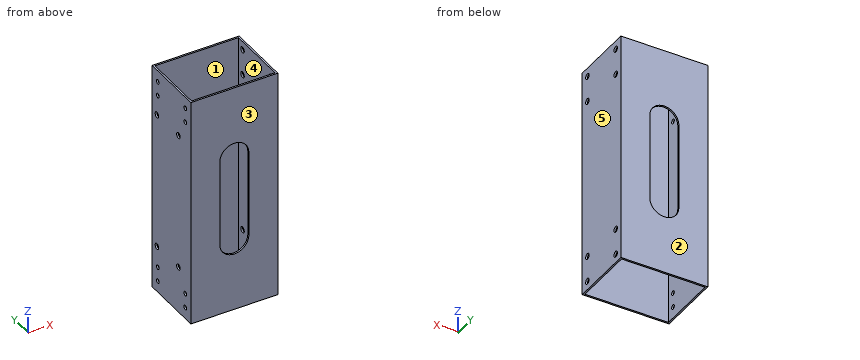
from build123d import *

# Parameters (mm, degrees)
SKETCH_1_W          = 60
SKETCH_1_H          = 45
SKETCH_1_W_2        = 57.6
SKETCH_1_H_2        = 42.6
EXTRUDE_1_DEPTH     = 80
SKETCH_4_R          = 2.025
CUT_EXTRUDE_1_DEPTH = 5
SKETCH_5_R          = 1.55
CUT_EXTRUDE_2_DEPTH = 5
SKETCH_6_R          = 2.025
CUT_EXTRUDE_3_DEPTH = 1.2
CUT_EXTRUDE_4_DEPTH = 160


with BuildPart() as part:
    # 草图1 → 凸台-拉伸1 (new body, symmetric)
    with BuildSketch(Plane.XY):
        Rectangle(SKETCH_1_W, SKETCH_1_H)
        Rectangle(SKETCH_1_W_2, SKETCH_1_H_2, mode=Mode.SUBTRACT)
    extrude(amount=EXTRUDE_1_DEPTH, both=True)

    # 草图4 → 切除-拉伸1 (cut, symmetric)
    with BuildSketch(Plane(origin=(30, 0, 0), x_dir=(0, 0, -1), z_dir=(1, 0, 0))):
        with Locations((-74, 16.5)):
            Circle(SKETCH_4_R)
        with Locations((-56, 16.5)):
            Circle(SKETCH_4_R)
        with Locations((-74, -16.5)):
            Circle(SKETCH_4_R)
        with Locations((-56, -16.5)):
            Circle(SKETCH_4_R)
    cut_extrude_1 = extrude(amount=CUT_EXTRUDE_1_DEPTH, both=True, mode=Mode.SUBTRACT)

    # 镜向1: 切除-拉伸1 across plane
    add(cut_extrude_1.mirror(Plane.XY), mode=Mode.SUBTRACT)

    # 草图5 → 切除-拉伸2 (cut, symmetric)
    with BuildSketch(Plane.ZY.offset(30)):
        with Locations((62, 16)):
            Circle(SKETCH_5_R)
        with Locations((72, 16)):
            Circle(SKETCH_5_R)
        with Locations((62, -16)):
            Circle(SKETCH_5_R)
        with Locations((72, -16)):
            Circle(SKETCH_5_R)
    cut_extrude_2 = extrude(amount=CUT_EXTRUDE_2_DEPTH, both=True, mode=Mode.SUBTRACT)

    # 镜向2: 切除-拉伸2 across plane
    add(cut_extrude_2.mirror(Plane.XY), mode=Mode.SUBTRACT)

    # 草图6 → 切除-拉伸3 (cut)
    with BuildSketch(Plane.ZY.offset(30)):
        with Locations((47.5, -8)):
            Circle(SKETCH_6_R)
        with Locations((47.5, 17)):
            Circle(SKETCH_6_R)
        with Locations((-47.5, 17)):
            Circle(SKETCH_6_R)
        with Locations((-47.5, -8)):
            Circle(SKETCH_6_R)
    extrude(amount=-CUT_EXTRUDE_3_DEPTH, mode=Mode.SUBTRACT)

    # 草图7 → 切除-拉伸4 (cut)
    with BuildSketch(Plane.XZ.offset(22.5)):
        with BuildLine():
            Line((-10, -30), (-10, 30))
            ThreePointArc((-10, 30), (0, 40), (10, 30))
            Line((10, 30), (10, -30))
            ThreePointArc((10, -30), (0, -40), (-10, -30))
        make_face()
    extrude(amount=-CUT_EXTRUDE_4_DEPTH, mode=Mode.SUBTRACT)


solid = part.part
The model under review builds one solid part; all positions refer to its coordinate system, in mm. Face numbers are marked on the shaded views. A direction names the side the tool comes from. Give positions to 0.01 mm unless a question says otherwise; leave off trailing zeros. Order: outer loops, then holes, each group sorted by start corner. A loop starts at its lowest first (then second) coordinate and runs counter-clockwise, first axis right, second up. Notation, with made-up numbers: (-36, 57) -> (-26, 57) arc R13 ccw to (-26, 61) -> close; hole circle Ø8 at (-32.5, -8.75). An arc over 180 degrees is marked (long way). Write item = value, one per line. Start each with the question number.
(1) Take a section at A-A (x = 0). Write out the cut boundary in (y, z).
(2) Draft analysis for pull direction X (two halves, no side actions). For the marked faces 3, 4 and 5, state which applies: +X half, -X half, draft (parallel to the pull), parting line (faces both ways), or undercut.
(3) Take a section at C-C (z = -52). Write out the cut boundary in (x, y).
(4) For pin 1 Ø2.5 at (y, z) = (-16, 72) entering from -X; pin 2 Ø3 at (y, z) = (-16.5, -74) entering from +X; pin 3 Ø5.5 at (y, z) = (17, -47.5) entering from -X, all flat-tipped, find the tip position at first contact; note any pin that passes through.
(5) Take a section at B-B (y = -1.5). Write out the cut boundary in (x, z).
(6) Tool access review of the marked faces 1 and 2: name each direction out of +Z, -Z, +X, -X, +Y, -Y from which nothing blocks a thin tool from reaching the whole face with its end or side.
(7) For L1, parallel to Y at x = 29, z = 56 (3 decimals); L2, parallel to X at y = 19, z = -42.5; L3, parallel to Y at x = -5, z = -55, list the stretches that pass through material, from the lowest coordinate up. Write a range as from..to.
(8) Take a section at D-D (x = 17.5). Write out the cut boundary in (y, z).
Returned:
q1.outline = (-22.5, -80) -> (-21.3, -80) -> (-21.3, -40) -> (-22.5, -40) -> close; (-22.5, 40) -> (-21.3, 40) -> (-21.3, 80) -> (-22.5, 80) -> close; (21.3, -80) -> (22.5, -80) -> (22.5, -40) -> (21.3, -40) -> close; (21.3, 40) -> (22.5, 40) -> (22.5, 80) -> (21.3, 80) -> close
q2.face_3 = draft
q2.face_4 = undercut
q2.face_5 = +X half
q3.outline = (-30, -22.5) -> (30, -22.5) -> (30, 22.5) -> (-30, 22.5) -> close; hole (-28.8, -21.3) -> (28.8, -21.3) -> (28.8, 21.3) -> (-28.8, 21.3) -> close
q4.pin_1 = 28.8
q4.pin_2 = -28.8
q4.pin_3 = -30
q5.outline = (-30, -80) -> (-28.8, -80) -> (-28.8, 80) -> (-30, 80) -> close; (28.8, -80) -> (30, -80) -> (30, 80) -> (28.8, 80) -> close
q6.face_1 = +Z, -Z
q6.face_2 = +Z, -Z, +X, -X, +Y
q7.L1 = -22.5..-18.525, -14.475..14.475, 18.525..22.5
q7.L2 = -30..-28.8, 28.8..30
q7.L3 = -22.5..-21.3, 21.3..22.5
q8.outline = (-22.5, -80) -> (-21.3, -80) -> (-21.3, 80) -> (-22.5, 80) -> close; (21.3, -80) -> (22.5, -80) -> (22.5, 80) -> (21.3, 80) -> close
